Can you work these out from the model? Positions are in its coordinate system, mm. Give positions to 0.01 mm unless a question says otherwise; leave off trailing zeros. Order: outer loops, then holes, each group sorted by start corner. A loop starts at its lowest first (then second) coordinate and runs counter-clockwise, first axis right, second up. Notation, with made-up numbers: (-22.75, 48) - (5.25, 48) arc R15 cw to (5.25, 64) - close; hole circle Ø5 at (-36, 18). An arc over 180 degrees is marked (long way). One line per question, with ' | ' between items.
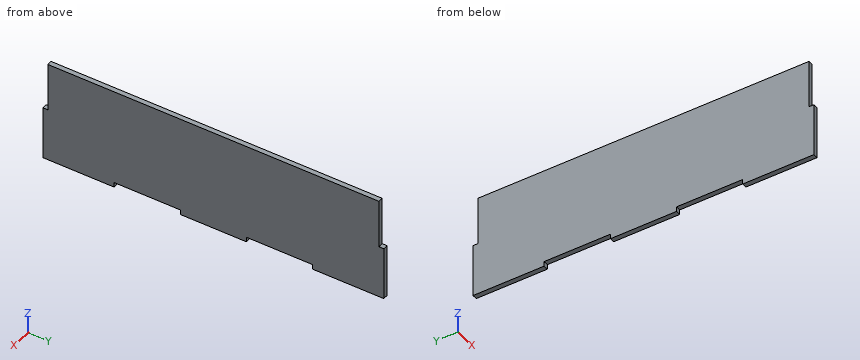
```python
from build123d import *

# Parameters (mm, degrees)
F0_W     = 73
F0_H     = 5
F0_W_2   = 5
F0_H_2   = 100
F1_DEPTH = 5


with BuildPart() as f1:
    # F0 (on Right) → F1 (new body)
    with BuildSketch(Plane.YZ):
        with Locations((138.5, -52.5)):
            Rectangle(F0_W, F0_H)
        Polygon((102, -50), (175, -50), (175, 0), (170, 0), (170, 50), (5, 50), (5, -50), (34, -50), align=None)
        Polygon((34, -55), (34, -50), (5, -50), (0, -50), (0, -55), align=None)
        with Locations((2.5, 0)):
            Rectangle(F0_W_2, F0_H_2)
        Polygon((0, -55), (0, -50), (-5, -50), (-34, -50), (-34, -55), align=None)
        with Locations((-2.5, 0)):
            Rectangle(F0_W_2, F0_H_2)
        Polygon((-34, -50), (-5, -50), (-5, 50), (-170, 50), (-170, 0), (-175, 0), (-175, -50), (-102, -50), align=None)
        with Locations((-138.5, -52.5)):
            Rectangle(F0_W, F0_H)
    extrude(amount=F1_DEPTH)


solid = f1.part
```
(1) Imagine slicing it at B-B (z = 15). List the corners of the cut face in (x, y) for me.
Answer below:
outline: (0, -170) - (5, -170) - (5, 170) - (0, 170) - close
(2) If I drill on line 1 (Y direction, x = 3.7, z = 15); line 2 (Z direction, x = 3.25, y = 86.5), over which ranges is the centre line in solid material (lowest first)?
Answer below:
line 1: -170 to 170 | line 2: -50 to 50
(3) Imagine slicing it at A-A (x = 3.7). List the corners of the cut face in (y, z) for me.
Answer below:
outline: (-175, -55) - (-102, -55) - (-102, -50) - (-34, -50) - (-34, -55) - (34, -55) - (34, -50) - (102, -50) - (102, -55) - (175, -55) - (175, 0) - (170, 0) - (170, 50) - (-170, 50) - (-170, 0) - (-175, 0) - close
(4) Will these pins go through, and if not, where does the flat tip stop? pin 1 (1 mm diameter, centred on x = 3.5, y = 80, fed in from -Z); pin 2 (2.5 mm diameter, centred on x = 2, z = 13.5, fed in from -Y); pin 3 (1 mm diameter, centred on x = 1, z = 31, fed in from +Y).
Answer below:
pin 1: z = -50 | pin 2: y = -170 | pin 3: y = 170
(5) Imagine slicing it at C-C (y = 67.5). List the corners of the cut face in (x, z) for me.
Answer below:
outline: (0, -50) - (5, -50) - (5, 50) - (0, 50) - close
